from build123d import *

# Parameters (mm, degrees)
SKETCH005_R     = 4.575
PAD002_DEPTH    = 1.55
SKETCH004_W     = 5
SKETCH004_H     = 5
PAD003_DEPTH    = 1.6
SKETCH006_R     = 1.7
POCKET001_DEPTH = 0.2
FILLET001_R     = 0.1


with BuildPart() as part:
    # Sketch005 → Pad002 (new body)
    with BuildSketch(Plane.XY):
        Circle(SKETCH005_R)
    extrude(amount=PAD002_DEPTH)

    # Sketch004 (on Face3 of Pad002) → Pad003 (join)
    with BuildSketch(Plane.XY.offset(1.55)):
        Rectangle(SKETCH004_W, SKETCH004_H)
    extrude(amount=PAD003_DEPTH)

    # Sketch006 (on Face8 of Pad003) → Pocket001 (cut)
    with BuildSketch(Plane.XY.offset(3.15)):
        Circle(SKETCH006_R)
    extrude(amount=-POCKET001_DEPTH, mode=Mode.SUBTRACT)

    # Fillet001
    fillet001_edges = [part.edges().sort_by_distance(p)[0] for p in [
        (-4.575, 0, 0),
        (-4.575, 0, 1.55),
    ]]
    fillet(fillet001_edges, radius=FILLET001_R)


with BuildPart() as part_1:
    # Body002 placement: moved
    add(part.part.moved(Location((0, -22, 0))))


solid = part_1.part
Work out the finished part from the listing and answer in its coordinate system (mm). A direction names the side the tool comes from. Give positions to 0.01 mm unless a question says otherwise; leave off trailing zeros. Loops run counter-clockwise (first coordinate to the right, second up) from the corner with the lowest first, then second, coordinate; pieces in that order, holes last. Notation, with made-up numbers: (10.5, 74.5) -> (63.5, 74.5) arc R20 ccw to (63.5, 112.5) -> close; hole circle Ø4 at (-38.5, 77). An arc over 180 degrees is marked (long way). Use a Markdown table: item, result. Add a question column.
1. Determine the mould class of faces 1 (the flat face through (0, -22, 2.95)), 2 (the flat face through (0, -19.5, 2)), 3 (the cylindrical face through (-0.992, -26.466, 0.766)) for opening direction X: released by +X, released by -X, zero draft, split by the parting line, or undercut.
2. Flat-ended cylindrical pins translate along their axes: pin 1 Ø0.8 at (x, z) = (-0.5, 2.5) entering from +Y; pin 2 Ø0.8 at (y, z) = (-21, 2.5) entering from -X; pin 3 Ø1.3 at (x, z) = (-1, 2) entering from -Y. Find the tip coordinate at first contact, or state that the pin passes through.
3. Section D-D on z = 1.2 is taken. Determine the outline of the cut face in (x, y) (3 decimals), and give its area (3 significant figures).
4. For faces 4 (the flat face through (0, -22, 0)), 5 (the flat face through (2.5, -22, 2)), 6 (the flat face through (-2.5, -22, 2)), 7 (the flat face through (0, -24.5, 2)), 8 (the flat face through (0, -20, 3.15)), determine the directions among +Z, -Z, +X, -X, +Y, -Y from which every point of the face is accessible in a straight line to the end or side of a thin tool.
5. Section B-B on y = -22 is taken. Determine the outline of the cut face in (x, z) (3 decimals), and give its area (3 significant figures).
6. Section C-C on z = 1.7 is taken. Determine the outline of the cut face in (x, y), and give its area (3 significant figures).
7. Section A-A on x = 0 is taken. Determine the outline of the cut face in (y, z) (3 decimals).
8. Find the intervals of material crossed by probe 1 along Y at (x, z) = (0, 3); probe 2 along X at (y, z) = (-24, 1.65); probe 3 along Y at (x, z) = (-1.25, 1.7), in increasing order.
Results below:
| question | item | result |
|---|---|---|
| 1 | face 1 | undercut |
| 1 | face 2 | zero draft |
| 1 | face 3 | split by the parting line |
| 2 | pin 1 | stops at y = -19.5 |
| 2 | pin 2 | stops at x = -2.5 |
| 2 | pin 3 | stops at y = -26.53 |
| 3 | outline | circle Ø9.15 at (0, -22) |
| 3 | area | 65.8 mm^2 |
| 4 | face 4 | -Z, +X, -X, +Y, -Y |
| 4 | face 5 | +Z, +X, +Y, -Y |
| 4 | face 6 | +Z, -X, +Y, -Y |
| 4 | face 7 | +Z, +X, -X, -Y |
| 4 | face 8 | +Z, +X, -X, +Y, -Y |
| 5 | outline | (-4.575, 0.1) arc R0.1 ccw to (-4.475, 0) -> (4.475, 0) arc R0.1 ccw to (4.575, 0.1) -> (4.575, 1.45) arc R0.1 ccw to (4.475, 1.55) -> (2.5, 1.55) -> (2.5, 3.15) -> (1.7, 3.15) -> (1.7, 2.95) -> (-1.7, 2.95) -> (-1.7, 3.15) -> (-2.5, 3.15) -> (-2.5, 1.55) -> (-4.475, 1.55) arc R0.1 ccw to (-4.575, 1.45) -> close |
| 5 | area | 21.5 mm^2 |
| 6 | outline | (-2.5, -24.5) -> (2.5, -24.5) -> (2.5, -19.5) -> (-2.5, -19.5) -> close |
| 6 | area | 25.0 mm^2 |
| 7 | outline | (-26.575, 0.1) arc R0.1 ccw to (-26.475, 0) -> (-17.525, 0) arc R0.1 ccw to (-17.425, 0.1) -> (-17.425, 1.45) arc R0.1 ccw to (-17.525, 1.55) -> (-19.5, 1.55) -> (-19.5, 3.15) -> (-20.3, 3.15) -> (-20.3, 2.95) -> (-23.7, 2.95) -> (-23.7, 3.15) -> (-24.5, 3.15) -> (-24.5, 1.55) -> (-26.475, 1.55) arc R0.1 ccw to (-26.575, 1.45) -> close |
| 8 | probe 1 | y = -24.5 to -23.7, -20.3 to -19.5 |
| 8 | probe 2 | x = -2.5 to 2.5 |
| 8 | probe 3 | y = -24.5 to -19.5 |
